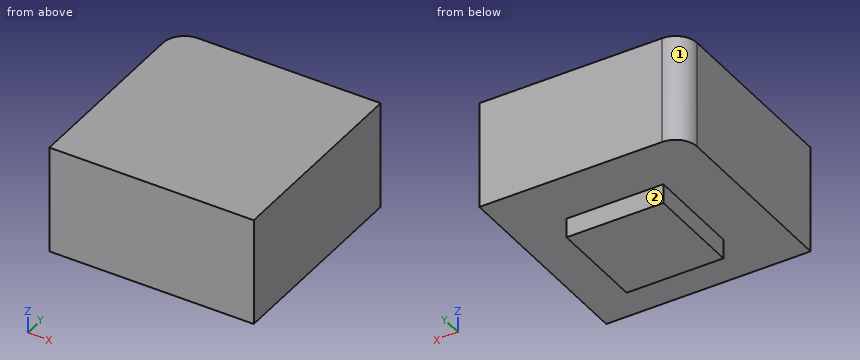
Autodesk Inventor part; units mm, degrees
ref_plane "YZ Plane" through (0, 0, 0) normal (1, 0, 0) x (0, 1, 0)
ref_plane "XZ Plane" through (0, 0, 0) normal (0, 1, 0) x (-1, 0, 0)
ref_plane "XY Plane" through (0, 0, 0) normal (0, 0, 1) x (1, 0, 0)
sketch "Esquisse1" plane through (0, 0, 0) normal (0, 0, 1) x (1, 0, 0)
  line L0 (0, -1.8) -> (0, 10.8)
  line L1 (-10.8, 0) -> (1.8, 0)
  line L2 (0, 0) -> (-9, 0)
  line L3 (-9, 0) -> (-9, 9)
  line L4 (-9, 9) -> (0, 9)
  line L5 (0, 9) -> (0, 0)
  point P0 (0, 9)
  dimension "d0" = 9
  dimension "d1" = 9
extrude "Extrusion1" add sketch "Esquisse1" along normal blind 1.8
sketch "Esquisse2" plane through (0, 0, 1.8) normal (0, 0, 1) x (1, 0, 0)
  line L0 (-14, 14) -> (5, 14)
  line L1 (5, 14) -> (5, -5)
  line L2 (5, -5) -> (-14, -5)
  line L3 (-14, -5) -> (-14, 14)
  line L4 (-9, 9) -> (-9, 0)
  line L5 (0, 9) -> (-9, 9)
  line L6 (0, 0) -> (0, 9)
  line L7 (-9, 0) -> (0, 0)
  dimension "d4" = 5
  dimension "d5" = 5
  dimension "d6" = 5
  dimension "d7" = 5
extrude "Extrusion2" add sketch "Esquisse2" along normal blind 10 contours L0 L1 L2 L3 | L5 L6 L7 L4
fillet "Congé1" radius 2 1 edges at (-14, 14, 6.8)
properties part number "pied_coque"
CAD build for the part. Positions are in the model's coordinates, mm. Face numbers are marked on the shaded views. A direction names the side the tool comes from. Coordinates: 2 decimals unless noted, no trailing zeros. Order: outer loops, then holes, each group sorted by start corner. A loop starts at its lowest first (then second) coordinate and runs counter-clockwise, first axis right, second up.
Item 1: Band-saw the part on C-C on z = 1. List the corners of the cut face in (x, y).
Check sheet entries:
outline: (-9, 0) - (0, 0) - (0, 9) - (-9, 9) - close
Item 2: Band-saw the part on D-D on x = 1. List the corners of the cut face in (y, z).
Check sheet entries:
outline: (-5, 1.8) - (14, 1.8) - (14, 11.8) - (-5, 11.8) - close
Item 3: Pin check, flat tips, straight feed: pin 1 Ø0.9 at (x, z) = (-2.5, 0.5) entering from -Y; pin 2 Ø0.5 at (x, z) = (-5, 0.5) entering from +Y; pin 3 Ø2 at (y, z) = (3.5, 0.5) entering from -X. Stop position of each tip, or through.
Check sheet entries:
pin 1: stops at y = 0
pin 2: stops at y = 9
pin 3: stops at x = -9
Item 4: Drill centre lines: L1, parallel to Z at x = -12.25, y = -3.75; L2, parallel to Y at x = -12.5, z = 3.5. Where is each one in solid material? Low to high.
Check sheet entries:
L1: z = 1.8 to 11.8
L2: y = -5 to 13.94
Item 5: 3-axis set-ups, long thin cutter, end or side, ignore diameter. For the marked faces 1 and 2: which of +Z, -Z, +X, -X, +Y, -Y reach the whole face in a straight line?
Check sheet entries:
face 1: +Z, -Z, -X, +Y
face 2: -Z, +X, -X, +Y
Item 6: Band-saw the part on B-B on y = 6.75. List the corners of the cut face in (x, z).
Check sheet entries:
outline: (-14, 1.8) - (-9, 1.8) - (-9, 0) - (0, 0) - (0, 1.8) - (5, 1.8) - (5, 11.8) - (-14, 11.8) - close
Item 7: Band-saw the part on A-A on x = -2.75. List the corners of the cut face in (y, z), plus the area to 3 significant figures.
Check sheet entries:
outline: (-5, 1.8) - (0, 1.8) - (0, 0) - (9, 0) - (9, 1.8) - (14, 1.8) - (14, 11.8) - (-5, 11.8) - close
area: 206 mm2
